```python
from build123d import *

# Parameters (mm, degrees)
SKETCH_1_R               = 22.5
SKETCH_1_R_2             = 9
EXTRUDE_1_DEPTH          = 3
SKETCH_2_R               = 1.6
CUT_EXTRUDE_1_DEPTH      = 4
PATTERN_CIRCULAR_2_COUNT = 4
SKETCH_3_R               = 11.25
SKETCH_3_R_2             = 9
CUT_EXTRUDE_2_DEPTH      = 1.5


with BuildPart() as part:
    # ｽｹｯﾁ1 → ﾎﾞｽ - 押し出し1 (new body)
    with BuildSketch(Plane.XY):
        Circle(SKETCH_1_R)
        Circle(SKETCH_1_R_2, mode=Mode.SUBTRACT)
    extrude(amount=EXTRUDE_1_DEPTH)

    # ｽｹｯﾁ2 → ｶｯﾄ - 押し出し1 (cut, through all)
    with BuildSketch(Plane.XY.offset(3)):
        with Locations((-17.5, 0)):
            Circle(SKETCH_2_R)
    cut_extrude_1 = extrude(amount=-CUT_EXTRUDE_1_DEPTH, mode=Mode.SUBTRACT)

    # 円形ﾊﾟﾀｰﾝ2: ｶｯﾄ - 押し出し1 ×4 about axis
    pattern_circular_2_axis = Axis((0, 0, 0), (0, 0, 1))
    for i in range(1, PATTERN_CIRCULAR_2_COUNT):
        add(cut_extrude_1.rotate(pattern_circular_2_axis, i * 360 / PATTERN_CIRCULAR_2_COUNT), mode=Mode.SUBTRACT)

    # ｽｹｯﾁ3 → ｶｯﾄ - 押し出し2 (cut)
    with BuildSketch(Plane.XY.offset(3)):
        Circle(SKETCH_3_R)
        Circle(SKETCH_3_R_2, mode=Mode.SUBTRACT)
    extrude(amount=-CUT_EXTRUDE_2_DEPTH, mode=Mode.SUBTRACT)


solid = part.part
```
Build history of the part. All positions in model axes, mm. A direction names the side the tool comes from. Give positions to 0.01 mm unless a question says otherwise; leave off trailing zeros. Loops run counter-clockwise (first coordinate to the right, second up) from the corner with the lowest first, then second, coordinate; pieces in that order, holes last.
Item 1: Drill centre lines: line 1 (Y direction, x = -5.5, z = 2.3); line 2 (X direction, y = 17.5, z = 0.75). Where is each one in solid material? Low to high.
Answers follow:
line 1: y = -21.82 to -9.81, 9.81 to 21.82
line 2: x = -14.14 to -1.6, 1.6 to 14.14
Item 2: Flat gauge pins, fed straight in: pin 1 (7 mm diameter, centred on x = 3, y = -4.5, fed in from +Z) (1 decimal); pin 2 (1 mm diameter, centred on x = -1.5, z = 2, fed in from +Y). Where does each tip first touch, or does it go through?
Answers follow:
pin 1: passes through
pin 2: stops at y = 22.48
Item 3: Slice it at C-C, the plane x = 17. List the corners of the cut face in (y, z), and give its area (3 significant figures).
Answers follow:
outline: (-14.74, 0) - (-1.52, 0) - (-1.52, 3) - (-14.74, 3) - close; (1.52, 0) - (14.74, 0) - (14.74, 3) - (1.52, 3) - close
area: 79.3 mm2
Item 4: Slice it at D-D, the plane y = 17.5. List the corners of the cut face in (x, z).
Answers follow:
outline: (-14.14, 0) - (-1.6, 0) - (-1.6, 3) - (-14.14, 3) - close; (1.6, 0) - (14.14, 0) - (14.14, 3) - (1.6, 3) - close
Item 5: Slice it at B-B, the plane z = 2.2. List the corners of the cut face in (x, y), and give its area (3 significant figures).
Answers follow:
outline: circle Ø45 at (0, 0); hole circle Ø3.2 at (-17.5, 0); hole circle Ø22.5 at (0, 0); hole circle Ø3.2 at (0, -17.5); hole circle Ø3.2 at (0, 17.5); hole circle Ø3.2 at (17.5, 0)
area: 1,160 mm2
Item 6: Pull direction X, two halves, no side cores. Call faces 3 (the face through (-5.3, 10.3, 3)), 4 (the face through (0.07, 19.1, 1.52)), 5 (the face through (10.382, -19.961, 1.479)): released by +X, released by -X, zero draft, split by the parting line, or undercut.
Answers follow:
face 3: zero draft
face 4: undercut
face 5: split by the parting line
Item 7: Which spindle directions (+Z, -Z, +X, -X, +Y, -Y) get a long thin tool onto all of the face, cutting with end or side? Do faces 1 (the face through (-5, 8, 1.5)), 2 (the face through (19.1, -0.07, 1.52)). Say none if no direction does.
Answers follow:
face 1: +Z
face 2: +Z, -Z
Item 8: Slice it at A-A, the plane x = 0. List the corners of the cut face in (y, z).
Answers follow:
outline: (-22.5, 0) - (-19.1, 0) - (-19.1, 3) - (-22.5, 3) - close; (-15.9, 0) - (-9, 0) - (-9, 1.5) - (-11.25, 1.5) - (-11.25, 3) - (-15.9, 3) - close; (9, 0) - (15.9, 0) - (15.9, 3) - (11.25, 3) - (11.25, 1.5) - (9, 1.5) - close; (19.1, 0) - (22.5, 0) - (22.5, 3) - (19.1, 3) - close
